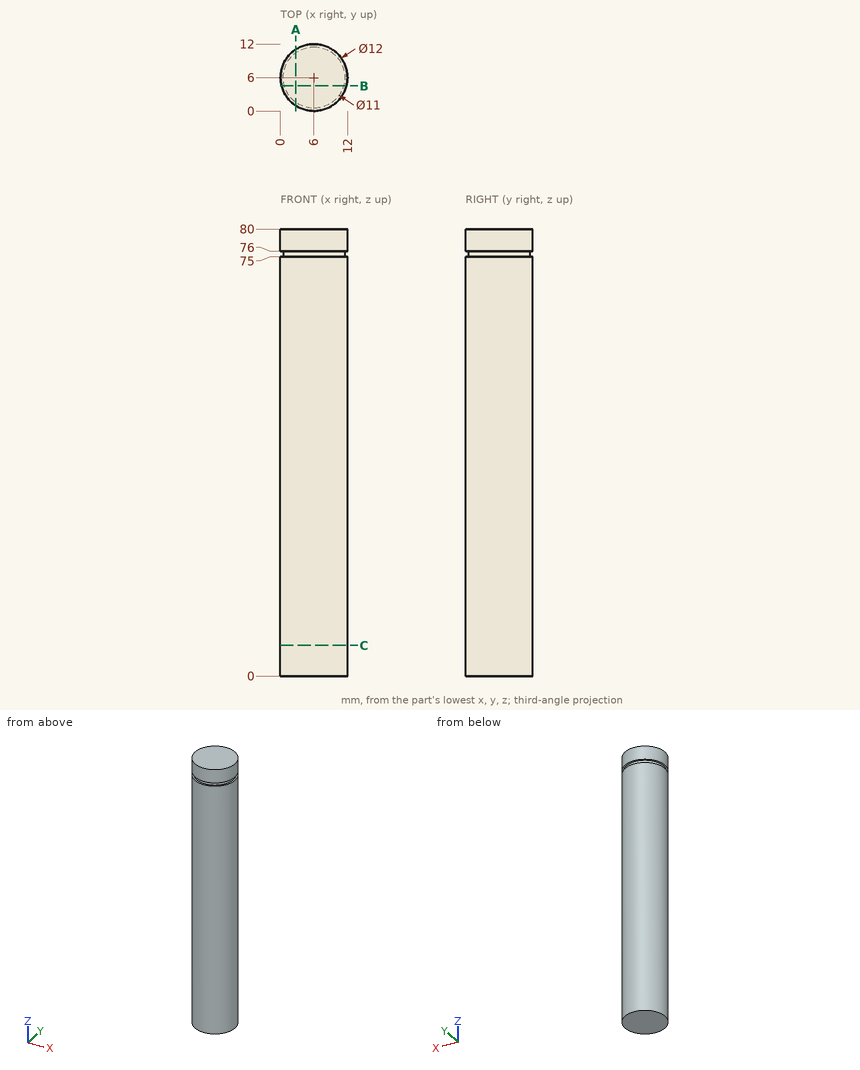
Source: three-view drawing plus pictorial views. Frame: mm from the lowest corner of the part. Round coordinates to 2 decimals unless told otherwise and drop trailing zeros. Loops run counter-clockwise (first coordinate to the right, second up) from the corner with the lowest first, then second, coordinate; pieces in that order, holes last. Notation, with made-up numbers: (67, 85) - (104, 85) arc R23 ccw to (104, 93) - close; hole circle Ø5 at (1.5, -12.75). An arc over 180 degrees is marked (long way). Write each question's results on one line, items separated by ' | '. Start each with the question number.
1) First-contact query: P1, Ø5, axis at x = 2, z = 30, coming from the +Y side; P2, Ø1, axis at y = 9.5, z = 48.5, coming from the -X side; P3, Ø1, axis at x = 9, z = 13.5, coming from the +Y side. Flat tips, straight axial feed; report the tip coordinate or a pass-through.
2) Cut plane A-A on x = 2.75. Return loops of the section in (y, z).
3) Cut plane B-B on y = 4.5. Return loops of the section in (x, z).
4) Line query: probe 1 along Y at (x, z) = (5.75, 70); probe 2 along Y at (x, z) = (11.5, 66); probe 3 along X at (y, z) = (5.5, 48). Output: solid intervals per line, ascending. Write a range as [from, to].
5) Cut plane C-C on z = 5.5. Return loops of the section in (x, y), then the cut area to 3 significant figures.
Verdict:
1) P1: stops at y = 11.81 | P2: stops at x = 0.8 | P3: stops at y = 11.45
2) outline: (0.96, 0) - (11.04, 0) - (11.04, 75) - (10.44, 75) - (10.44, 76) - (11.04, 76) - (11.04, 80) - (0.96, 80) - (0.96, 76) - (1.56, 76) - (1.56, 75) - (0.96, 75) - close
3) outline: (0.19, 0) - (11.81, 0) - (11.81, 75) - (11.29, 75) - (11.29, 76) - (11.81, 76) - (11.81, 80) - (0.19, 80) - (0.19, 76) - (0.71, 76) - (0.71, 75) - (0.19, 75) - close
4) probe 1: y = [0.01, 11.99] | probe 2: y = [3.6, 8.4] | probe 3: x = [0.02, 11.98]
5) outline: circle Ø12 at (6, 6) | area: 113 mm2
